from build123d import *

# Parameters (mm, degrees)
BOSS_EXTRUDE1_DEPTH = 20
SKETCH3_R           = 6
CUT_EXTRUDE1_DEPTH  = 115.891252931


with BuildPart() as part:
    # Sketch2 → Boss-Extrude1 (new body)
    with BuildSketch(Plane.XY):
        with BuildLine():
            Line((28, 72.747460854), (28, 80))
            Line((28, 80), (52, 80))
            Line((52, 80), (52, 72.747460854))
            ThreePointArc((52, 72.747460854), (52.659356425, 70.547438013), (54.420050252, 69.072714769))
            ThreePointArc((54.420050252, 69.072714769), (69.23734115, 57.280554554), (76.020050252, 39.6))
            ThreePointArc((76.020050252, 39.6), (77.316718427, 37.033520605), (80, 36))
            Line((80, 36), (80, 0))
            Line((80, 0), (64, 0))
            Line((64, 0), (64, 12))
            Line((64, 12), (70, 12))
            Line((70, 12), (70, 36))
            Line((70, 36), (64.200502516, 36))
            ThreePointArc((64.200502516, 36), (57.100028243, 53.041303653), (40, 59.999162459))
            ThreePointArc((40, 59.999162459), (22.899971757, 53.041303653), (15.799497484, 36))
            Line((15.799497484, 36), (10, 36))
            Line((10, 36), (10, 12))
            Line((10, 12), (16, 12))
            Line((16, 12), (16, 0))
            Line((16, 0), (0, 0))
            Line((0, 0), (0, 36))
            ThreePointArc((0, 36), (2.683281573, 37.033520605), (3.979949748, 39.6))
            ThreePointArc((3.979949748, 39.6), (10.76265885, 57.280554554), (25.579949748, 69.072714769))
            ThreePointArc((25.579949748, 69.072714769), (27.340643575, 70.547438013), (28, 72.747460854))
        make_face()
    extrude(amount=-BOSS_EXTRUDE1_DEPTH)

    # Sketch3 → Cut-Extrude1 (cut, through all)
    with BuildSketch(Plane(origin=(0, 80, 0), x_dir=(1, 0, 0), z_dir=(0, 1, 0))):
        with Locations(Location((40, 10, 0), (0, 0, 270))):
            Circle(SKETCH3_R)
    extrude(amount=-CUT_EXTRUDE1_DEPTH, mode=Mode.SUBTRACT)


solid = part.part
Here's how the part is built. I have some questions about the finished solid (model axes, mm). A direction names the side the tool comes from. Coordinates: 2 decimals unless noted, no trailing zeros. Order: outer loops, then holes, each group sorted by start corner. A loop starts at its lowest first (then second) coordinate and runs counter-clockwise, first axis right, second up. Notation, with made-up numbers: (78, 43) -> (100, 43) arc R28 ccw to (100, 67) -> close; hole circle Ø8 at (45, -17). An arc over 180 degrees is marked (long way). Answer in a Markdown table with one row per item.
(1) On a 3-axis mill with a long thin cutter (end or side, diameter ignored), from which of +Z, -Z, +X, -X, +Y, -Y can I reach the whole of each face in a straight line? I mean faces 1 (the face through (10, 24, -10)), 2 (the face through (28, 76, -10)), 3 (the face through (52, 76, -10)). Say none if no direction works.
Answer key:
| item | result |
|---|---|
| face 1 | +Z, -Z |
| face 2 | +Z, -Z, -X, +Y |
| face 3 | +Z, -Z, +X, +Y |
(2) Thinking about a two-plate mould opening in X: for faces 4 (the face through (72, 0, -10)), 5 (the face through (13, 12, -10)), 6 (the face through (10.6, 57.06, -9.86)), which applies, +X half, -X half, draft (parallel to the pull), parting line (faces both ways), or undercut?
Answer key:
| item | result |
|---|---|
| face 4 | draft |
| face 5 | undercut |
| face 6 | -X half |
(3) Will these pins go through, and if not, where does the flat tip stop? pin 1 Ø6 at (x, z) = (57, -14) entering from -Y; pin 2 Ø3.5 at (y, z) = (75, -15) entering from +X; pin 3 Ø12 at (y, z) = (43, -12) entering from +X.
Answer key:
| item | result |
|---|---|
| pin 1 | y = 49.56 |
| pin 2 | x = 52 |
| pin 3 | x = 77.35 |
(4) Please list where these lines run through material, in increasing order: probe 1 along X at (y, z) = (12.5, -11.75); probe 2 along Z at (x, y) = (40, 70.5); probe 3 along X at (y, z) = (74, -10).
Answer key:
| item | result |
|---|---|
| probe 1 | 0 to 10, 70 to 80 |
| probe 2 | -20 to -16, -4 to 0 |
| probe 3 | 28 to 34, 46 to 52 |
(5) I want a section at C-C on y = 6. List the corners of the cut face in (x, z) for me, then the cut area to 3 significant figures.
Answer key:
| item | result |
|---|---|
| outline | (0, -20) -> (16, -20) -> (16, 0) -> (0, 0) -> close; (64, -20) -> (80, -20) -> (80, 0) -> (64, 0) -> close |
| area | 640 mm^2 |
(6) I want a section at D-D on x = 13.5. List the corners of the cut face in (y, z) for me, then the cut area to 3 significant figures.
Answer key:
| item | result |
|---|---|
| outline | (0, -20) -> (12, -20) -> (12, 0) -> (0, 0) -> close; (36, -20) -> (60.58, -20) -> (60.58, 0) -> (36, 0) -> close |
| area | 732 mm^2 |
(7) I want a section at A-A on z = -10. List the corners of the cut face in (x, y) for me, then the cut area to 3 significant figures.
Answer key:
| item | result |
|---|---|
| outline | (0, 0) -> (16, 0) -> (16, 12) -> (10, 12) -> (10, 36) -> (15.8, 36) arc R24 cw to (34, 59.29) -> (34, 80) -> (28, 80) -> (28, 72.75) arc R4 cw to (25.58, 69.07) arc R36 ccw to (3.98, 39.6) arc R4 cw to (0, 36) -> close; (46, 59.29) arc R24 cw to (64.2, 36) -> (70, 36) -> (70, 12) -> (64, 12) -> (64, 0) -> (80, 0) -> (80, 36) arc R4 cw to (76.02, 39.6) arc R36 ccw to (54.42, 69.07) arc R4 cw to (52, 72.75) -> (52, 80) -> (46, 80) -> close |
| area | 1,970 mm^2 |
(8) I want a section at B-B on y = 74.5. List the corners of the cut face in (x, z) for me.
Answer key:
| item | result |
|---|---|
| outline | (28, -20) -> (52, -20) -> (52, 0) -> (28, 0) -> close; hole circle Ø12 at (40, -10) |
